Here's how the part is built. I have some questions about the finished solid (model axes, mm). Face numbers are marked on the shaded views. A direction names the side the tool comes from. Give positions to 0.01 mm unless a question says otherwise; leave off trailing zeros. Loops run counter-clockwise (first coordinate to the right, second up) from the corner with the lowest first, then second, coordinate; pieces in that order, holes last. Notation, with made-up numbers: (31, -36) -> (75, -36) arc R15 cw to (75, -17) -> close; hole circle Ø8 at (-2, -35.75). An arc over 180 degrees is marked (long way). Answer in a Markdown table with one row per item. Add a question column.
Item 1: If we section it at A-A (x = 87.5): Write out the boundary of the cut face in (y, z).
Item 2: Which directions (+Z, -Z, +X, -X, +Y, -Y) give clear straight access to the entire face, cutting with the end or side of a thin tool? Please do the marked faces 1 and 2.
Item 3: If I drill on line 1 (Z direction, x = 43.5, y = 0.5); line 2 (X direction, y = 7, z = 4); line 3 (Y direction, x = 10, z = 0.25), over which ranges is the centre line in solid material (lowest first)?
Item 4: For P1, Ø4, axis at y = 9.5, z = 9, coming from the +X side; P2, Ø6, axis at x = 36, z = -0.5, coming from the +Y side; P3, Ø5, axis at x = 66, y = 3, coming from the -Z side, each with a flat end and sliding along its axis, tell me the tip position at first contact or that it passes through.
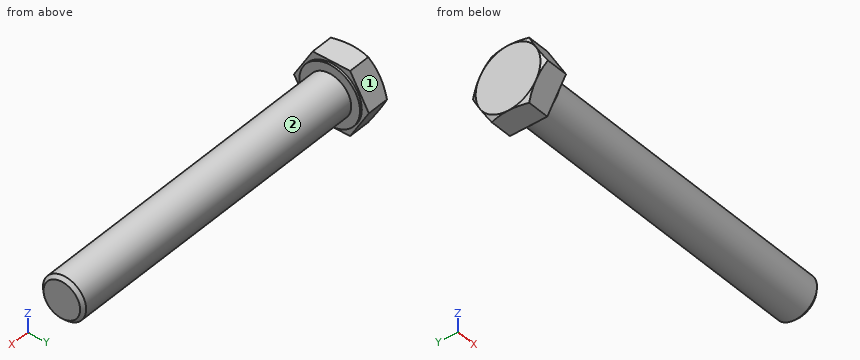
Autodesk Inventor part; units mm, degrees
ref_plane "Work Plane1" through (1.525, 0, 0) normal (0, 0, 1) x (1, 0, 0)
ref_plane "YZ Plane" through (0, 0, 0) normal (1, 0, 0) x (0, 1, 0)
ref_plane "XZ Plane" through (0, 0, 0) normal (0, 1, 0) x (-1, 0, 0)
sketch "Sketch1" plane through (0, 0, 0) normal (0, 0, 1) x (1, 0, 0)
  line L0 (0, 11.245) -> (0, 8)
  line L1 (6, 8) -> (120, 8)
  line L2 (120, 8) -> (120, 0)
  line L3 (120, 0) -> (-0.8001, 0)
  line L4 (-24.9601, 0) -> (144.16, 0)
  line L5 (-0.8001, 0) -> (-0.8001, 11.245)
  line L6 (-0.8001, 11.245) -> (0, 11.245)
  line L7 (6, 8) -> (4.773, 8)
  line L8 (4.773, 8) -> (0, 8)
  line L9 (0, -2.249) -> (0, 13.494)
  dimension "d0" = 120
  dimension "d1" = 114
  dimension "d2" = 16
  dimension "d9" = 0.8001
  dimension "d10" = 22.49
  dimension "d13" = 1.227
  dimension "d14" = 16
revolve "Body" add sketch "Sketch1" angle 360 about axis through (120, 0, 0) along (-1, 0, 0)
sketch "Sketch2" plane through (-0.8001, 0, 0) normal (-1, 0, 0) x (0, 0, 1)
  line L0 (0, 13.8564) -> (12, 6.9282)
  line L1 (12, 6.9282) -> (12, -6.9282)
  line L2 (12, -6.9282) -> (0, -13.8564)
  line L3 (0, -13.8564) -> (-12, -6.9282)
  line L4 (-12, -6.9282) -> (-12, 6.9282)
  line L5 (-12, 6.9282) -> (0, 13.8564)
  point P0 (0, 0)
  point P1 (0, 0)
  dimension "d11" = 24
extrude "Head" add sketch "Sketch2" along normal blind 9.2
sketch "Sketch4" plane through (0, 0, 0) normal (0, 0, 1) x (1, 0, 0)
  line L0 (-10.0001, 12) -> (-10.0001, 13.8564)
  line L1 (-10.0001, 13.8564) -> (-8.9283, 13.8564)
  line L2 (-8.9283, 13.8564) -> (-10.0001, 12)
  line L3 (-11.8401, 0) -> (1.0399, 0)
  line L4 (-0.8001, 13.8564) -> (-10.0001, 13.8564)
  line L5 (-10.0001, 6.9282) -> (-10.0001, 13.8564)
  dimension "d5" = 30
  dimension "d19" = 24
revolve "Chamfer1" cut sketch "Sketch4" angle 360 about axis through (-10, 0, 0) along (1, 0, 0)
thread "Thread"
chamfer "Chamfer2" distance 1.2269 distance2 1.227 1 edges at (120, -8, 0) measured on face at (120, 0.8907, 2.0408)
ref_plane "Work Plane1" through (1.525, 0, 0) normal (0, 0, 1) x (1, 0, 0)
equation "\"d0\" = NLG"
equation "\"d1\" = GEL"
equation "\"d2\" = GD"
equation "\"d10\" = SD2"
equation "\"d14\" = BDM"
equation "\"d11\" = SW"
equation "\"d3\" = KOH - SD"
equation "\"d5\" = ANG1"
equation "\"d19\" = SW0"
equation "\"d15\" = GEL"
equation "\"d6\" = -0.5 * SPD + 0.5 * GD"
equation "\"NLG\" = 120"
equation "\"GD\" = NND"
equation "\"BDM\" = NND"
equation "\"KOH\" = 10"
equation "\"GEL\" = 114"
equation "\"SW\" = 24"
equation "\"SW0\" = SW"
equation "\"SPD\" = NND - 1.2269 * PTC"
equation "\"SD2\" = 22.49"
equation "\"SD\" = 0.8"
equation "\"ANG1\" = 30deg"
equation "\"GAL\" = 0.61345 * PTC"
equation "\"GUL\" = 0.61345 * PTC"
equation "\"RR\" = 0.6"
equation "\"GD1\" = THREADDIA - 1.2269 * PTC"
equation "\"THREADDIA\" = 16"
equation "\"SDH\" = SD2"
equation "\"SDHG\" = 6"
equation "\"TOA\" = 30deg"
equation "\"PTC\" = 2"
equation "\"NND\" = 16"
equation "\"E0\" = 27.72"
properties part number "ISO 4017 - M16 x 120" material "Steel, Mild"
Recorded:
| question | item | result |
|---|---|---|
| 1 | outline | circle Ø16 at (0, 0) |
| 2 | face 1 | +Z, +X, -X, +Y |
| 2 | face 2 | +X |
| 3 | line 1 | z = -7.98 to 7.98 |
| 3 | line 2 | x = -10 to 0 |
| 3 | line 3 | y = -8 to 8 |
| 4 | P1 | stops at x = 0 |
| 4 | P2 | stops at y = 8 |
| 4 | P3 | stops at z = -7.98 |
